Read the model definition and answer for the solid it produces. Units are mm, in the model's axes. A direction names the side the tool comes from. Coordinates: 2 decimals unless noted, no trailing zeros. Order: outer loops, then holes, each group sorted by start corner. A loop starts at its lowest first (then second) coordinate and runs counter-clockwise, first axis right, second up.
```python
from build123d import *

# Parameters (mm, degrees)
F0_R     = 20
F1_DEPTH = 10
F3_DEPTH = 6
F4_SIZE2 = 5
F4_SIZE  = 6
F5_R     = 4


with BuildPart() as f1:
    # F0 (on Top) → F1 (new body)
    with BuildSketch(Plane.XY):
        Circle(F0_R)
    extrude(amount=F1_DEPTH)

    # F2 (on face) → F3 (cut)
    with BuildSketch(Plane.XY.offset(10)):
        Polygon((3.0022213998, -5.2), (6.0044427996, 0), (3.0022213998, 5.2), (-3.0022213998, 5.2), (-6.0044427996, 0), (-3.0022213998, -5.2), align=None)
    extrude(amount=-F3_DEPTH, mode=Mode.SUBTRACT)

    # F4
    f4_edges = [f1.edges().sort_by_distance(p)[0] for p in [
        (-20, 0, 10),
    ]]
    f4_side = f1.faces().sort_by_distance((-19.434315, 0, 10))[0]
    chamfer(f4_edges, length=F4_SIZE, length2=F4_SIZE2, reference=f4_side)

    # F5
    f5_edges = [f1.edges().sort_by_distance(p)[0] for p in [
        (-14, 0, 10),
        (-20, 0, 5),
    ]]
    fillet(f5_edges, radius=F5_R)


solid = f1.part
```
1) Straight lines are drawn through the part: line 1 (X direction, y = -3, z = 8); line 2 (Y direction, x = -5.5, z = 7.25); line 3 (Y direction, x = -1.5, z = 5.75). For each, find the intervals that lie inside material, in ascending order.
A:
line 1: x = -16.12 to -4.27, 4.27 to 16.12
line 2: y = -16.4 to -0.87, 0.87 to 16.4
line 3: y = -18.96 to -5.2, 5.2 to 18.96
2) Flat-ended cylindrical pins translate along their axes: pin 1 Ø4 at (x, z) = (9.5, 4.5) entering from -Y; pin 2 Ø1.8 at (x, z) = (1, 8.5) entering from -Y; pin 3 Ø1.5 at (y, z) = (3.5, 7) entering from +X. Find the tip coordinate at first contact, or state that the pin passes through.
A:
pin 1: stops at y = -18.43
pin 2: stops at y = -16.85
pin 3: stops at x = 18.18
3) A cutting plane is placed at A-A, the plane z = 8. Determine the outline of the cut face in (x, y), and give its area (3 significant figures).
A:
outline: circle Ø32.8 at (0, 0); hole (-6, 0) - (-3, -5.2) - (3, -5.2) - (6, 0) - (3, 5.2) - (-3, 5.2) - close
area: 751 mm2
4) A cutting plane is placed at B-B, the plane z = 0.5. Determine the outline of the cut face in (x, y).
A:
outline: circle Ø40 at (0, 0)
5) Determine the mould class of faces 1 (the flat face through (-0.2, -5.4, 10)), 2 (the flat face through (4.524, 2.564, 7.042)), 3 (the conical face through (14.62, 4.604, 8.893)) for opening direction Y: pulls with the +Y half, pulls with the -Y half, needs draft (parallel to the pull), parting line crosses it, or undercut.
A:
face 1: needs draft
face 2: undercut
face 3: parting line crosses it
6) Which of the six approach directions +Z, -Z, +X, -X, +Y, -Y give full straight-line access (tool end or side, diameter ignored) to faces 4 (the flat face through (4.48, -2.64, 7.04)), 5 (the flat face through (0, 0, 0))?
A:
face 4: +Z
face 5: -Z, +X, -X, +Y, -Y
